from build123d import *

# Parameters (mm, degrees)
SKETCH1_W                      = 40
SKETCH1_H                      = 60
BOSS_EXTRUDE1_DEPTH            = 40
SKETCH2_W                      = 52
SKETCH2_H                      = 24
CUT_EXTRUDE1_DEPTH             = 83.462112512
F_4_5_4_5_DIAMETER_HOLE1_D     = 4.5
F_22_0_22_DIAMETER_HOLE2_D     = 22
F_22_0_22_DIAMETER_HOLE2_DEPTH = 7
F_22_0_22_DIAMETER_HOLE1_D     = 22
F_22_0_22_DIAMETER_HOLE1_DEPTH = 7
F_2_5_2_5_DIAMETER_HOLE1_D     = 2.5
F_2_5_2_5_DIAMETER_HOLE1_DEPTH = 8
F_2_5_2_5_DIAMETER_HOLE1_TIP   = 0.721687836
CHAMFER1_SIZE                  = 2
F_19_0_19_DIAMETER_HOLE1_D     = 19
F_2MM_PIN_REACH                = 78.837
SKETCH13_R                     = 1


with BuildPart() as part:
    # Sketch1 → Boss-Extrude1 (new body)
    with BuildSketch(Plane(origin=(0, 40, 0), x_dir=(1, 0, 0), z_dir=(0, 1, 0))):
        with Locations((20, -30)):
            Rectangle(SKETCH1_W, SKETCH1_H)
    extrude(amount=-BOSS_EXTRUDE1_DEPTH)

    # Sketch2 → Cut-Extrude1 (cut, through all)
    with BuildSketch(Plane(origin=(40, 0, 0), x_dir=(0, 0, -1), z_dir=(1, 0, 0))):
        with Locations((-34, 20)):
            Rectangle(SKETCH2_W, SKETCH2_H)
    extrude(amount=-CUT_EXTRUDE1_DEPTH, mode=Mode.SUBTRACT)

    # Ø4.5 (4.5) Diameter Hole1 (through all)
    with Locations(Plane.XY.offset(8)):
        with Locations((20, 20)):
            Hole(F_4_5_4_5_DIAMETER_HOLE1_D / 2)

    # Ø22.0 (22) Diameter Hole2
    with Locations(Plane(origin=(0, 40, 0), x_dir=(-1, 0, 0), z_dir=(0, 1, 0))):
        with Locations((-20, 35)):
            Hole(F_22_0_22_DIAMETER_HOLE2_D / 2, depth=F_22_0_22_DIAMETER_HOLE2_DEPTH)

    # Ø22.0 (22) Diameter Hole1
    with Locations(Plane.XZ):
        with Locations((20, 35)):
            Hole(F_22_0_22_DIAMETER_HOLE1_D / 2, depth=F_22_0_22_DIAMETER_HOLE1_DEPTH)

    # Ø2.5 (2.5) Diameter Hole1
    with Locations(Plane(origin=(0, 40, 0), x_dir=(1, 0, 0), z_dir=(0, 1, 0))):
        with Locations((33.24990566, -16.2), (6.75009434, -53.8)):
            Hole(F_2_5_2_5_DIAMETER_HOLE1_D / 2, depth=F_2_5_2_5_DIAMETER_HOLE1_DEPTH)
            with Locations((0, 0, -(F_2_5_2_5_DIAMETER_HOLE1_DEPTH + F_2_5_2_5_DIAMETER_HOLE1_TIP / 2))):  # 120° drill point
                Cone(0, F_2_5_2_5_DIAMETER_HOLE1_D / 2, F_2_5_2_5_DIAMETER_HOLE1_TIP, mode=Mode.SUBTRACT)

    # Chamfer1
    chamfer1_edges = [part.edges().sort_by_distance(p)[0] for p in [
        (22.25, 20, 8),
    ]]
    chamfer(chamfer1_edges, length=CHAMFER1_SIZE)

    # Ø19.0 (19) Diameter Hole1 (through all)
    with Locations(Plane(origin=(0, 7, 0), x_dir=(-1, 0, 0), z_dir=(0, -1, 0))):
        with Locations((-20, -35)):
            Hole(F_19_0_19_DIAMETER_HOLE1_D / 2)

    # Sketch13 → 2mm Pin (cut, up to next)
    with BuildSketch(Plane.XY.offset(8), mode=Mode.PRIVATE) as f_2mm_pin_sk1:
        with Locations((10, 20)):
            Circle(SKETCH13_R)
    f_2mm_pin_tool1 = extrude(f_2mm_pin_sk1.sketch, amount=-F_2MM_PIN_REACH, mode=Mode.PRIVATE) & part.part
    add(f_2mm_pin_tool1.solids().sort_by_distance((10, 20, 8))[0], mode=Mode.SUBTRACT)


solid = part.part
Can you work these out from the model? Positions are in its coordinate system, mm. A direction names the side the tool comes from. Round coordinates to 2 decimals unless told otherwise and drop trailing zeros. Order: outer loops, then holes, each group sorted by start corner. A loop starts at its lowest first (then second) coordinate and runs counter-clockwise, first axis right, second up. Notation, with made-up numbers: (-10.5, 45.25) -> (-3.5, 45.25) arc R13 ccw to (-3.5, 64.25) -> close; hole circle Ø7 at (-25.5, 31). An arc over 180 degrees is marked (long way). Write each question's results on one line, items separated by ' | '. Start each with the question number.
Item 1: Which directions (+Z, -Z, +X, -X, +Y, -Y) give clear straight access to the entire face, cutting with the end or side of a thin tool? Please do faces 1 (the flat face through (20, 0, 23)), 2 (the flat face through (0, 34, 30)), 3 (the cylindrical face through (9.508, 3.549, 38.304)), 4 (the flat face through (10, 33, 35)), 5 (the flat face through (11, 32, 40)).
Item 2: Thinking about a two-plate mould opening in Z: for faces 6 (the flat face through (24, 20, 0)), 7 (the cylindrical face through (32.095, 35.944, 16.679)), 8 (the flat face through (20, 4, 60)), 9 (the cylindrical face through (10, 19, 4)), which applies, +Z half, -Z half, draft (parallel to the pull), parting line (faces both ways), or undercut?
Item 3: If we section it at B-B, the plane x = 20: State how many separate pieces and enclosed holes the cut face has, then the cut area to 3 significant figures.
Item 4: Please list where these lines run through material, in increasing order: L1, parallel to Y at x = 26.5, z = 17; L2, parallel to Z at x = 20, y = 7.5; L3, parallel to X at y = 34.5, z = 53.8.
Item 5: Will these pins go through, and if not, where does the flat tip stop? pin 1 (2.5 mm diameter, centred on x = 10, y = 20, fed in from +Z); pin 2 (5 mm diameter, centred on x = 20, y = 20, fed in from +Z).
Item 6: If we section it at A-A, the plane z = 35: Write out the boundary of the cut face in (x, y).
Item 7: If we section it at C-C, the plane z = 16.2: Write out the boundary of the cut face in (x, y), then the cut area to 3 significant figures.
Item 8: If we section it at D-D, the plane y = 20: Write out the boundary of the cut face in (x, z).
Results:
1) face 1: +Z, -Z, +X, -X, -Y | face 2: +Z, -Z, -X, +Y, -Y | face 3: -Y | face 4: +Y | face 5: +Z, +X, -X
2) face 6: -Z half | face 7: undercut | face 8: +Z half | face 9: draft
3) separate pieces: 4 | enclosed holes: 0 | area: 766 mm2
4) L1: y = 0 to 8, 32 to 40 | L2: z = 0 to 25.5, 44.5 to 60 | L3: x = 0 to 5.5, 8 to 40
5) pin 1: stops at z = 8 | pin 2: stops at z = 6.25
6) outline: (0, 0) -> (9, 0) -> (9, 7) -> (10.5, 7) -> (10.5, 8) -> (0, 8) -> close; (0, 32) -> (10.5, 32) -> (10.5, 33) -> (9, 33) -> (9, 40) -> (0, 40) -> close; (29.5, 7) -> (31, 7) -> (31, 0) -> (40, 0) -> (40, 8) -> (29.5, 8) -> close; (29.5, 32) -> (40, 32) -> (40, 40) -> (31, 40) -> (31, 33) -> (29.5, 33) -> close
7) outline: (0, 0) -> (40, 0) -> (40, 8) -> (0, 8) -> close; (0, 32) -> (32, 32) -> (32, 40) -> (0, 40) -> close; (34.5, 32) -> (40, 32) -> (40, 40) -> (34.5, 40) -> close | area: 620 mm2
8) outline: (0, 0) -> (9, 0) -> (9, 8) -> (0, 8) -> close; (11, 0) -> (17.75, 0) -> (17.75, 6) -> (15.75, 8) -> (11, 8) -> close; (22.25, 0) -> (40, 0) -> (40, 8) -> (24.25, 8) -> (22.25, 6) -> close
